from build123d import *

# Parameters (mm, degrees)
SKETCH1_R           = 25
BOSS_EXTRUDE1_DEPTH = 17
CIRPATTERN1_COUNT   = 3
SKETCH14_W          = 15.649879363
SKETCH14_H          = 14
CUT_EXTRUDE2_DEPTH  = 17.25
CUT_EXTRUDE3_DEPTH  = 15
SKETCH16_R          = 2
SKETCH16_R_2        = 1
BOSS_EXTRUDE2_DEPTH = 3


with BuildPart() as part:
    # Sketch1 → Boss-Extrude1 (new body)
    with BuildSketch(Plane.XY):
        Circle(SKETCH1_R)
    extrude(amount=BOSS_EXTRUDE1_DEPTH)

    # Sketch12 → Ø3.0mm Dowel Hole1 (revolve, cut)
    with BuildSketch(Plane(origin=(0, 21, 0), x_dir=(0, 1, 0), z_dir=(1, 0, 0))):
        Polygon((0, 0), (0, 5.901290929), (1.5, 5), (1.5, 0), align=None)
    f_3_0mm_dowel_hole1 = revolve(axis=Axis((0, 21, -6.35), (0, 0, 1)), mode=Mode.SUBTRACT)

    # CirPattern1: Ø3.0mm Dowel Hole1 ×3 about axis
    cirpattern1_axis = Axis((0, 0, 0), (0, 0, 1))
    for i in range(1, CIRPATTERN1_COUNT):
        add(f_3_0mm_dowel_hole1.rotate(cirpattern1_axis, i * 360 / CIRPATTERN1_COUNT), mode=Mode.SUBTRACT)

    # Sketch14 → Cut-Extrude2 (cut)
    with BuildSketch(Plane(origin=(0, -25, 0), x_dir=(-1, 0, 0), z_dir=(0, -1, 0))):
        with Locations((-0.842506508, -8.397851159)):
            Rectangle(SKETCH14_W, SKETCH14_H)
    extrude(amount=-CUT_EXTRUDE2_DEPTH, mode=Mode.SUBTRACT)

    # Sketch15 → Cut-Extrude3 (cut)
    with BuildSketch(Plane(origin=(0, 0, 0), x_dir=(-1, 0, 0), z_dir=(0, 0, -1))):
        with BuildLine():
            ThreePointArc((-3.981818088, 20.619047619), (0, 17), (3.981818088, 20.619047619))
            ThreePointArc((3.981818088, 20.619047619), (18.186533479, 10.5), (19.847528084, -6.861168192))
            ThreePointArc((19.847528084, -6.861168192), (14.722431864, -8.5), (15.865709996, -13.757879427))
            ThreePointArc((15.865709996, -13.757879427), (0, -21), (-15.865709996, -13.757879427))
            ThreePointArc((-15.865709996, -13.757879427), (-14.722431864, -8.5), (-19.847528084, -6.861168192))
            ThreePointArc((-19.847528084, -6.861168192), (-18.186533479, 10.5), (-3.981818088, 20.619047619))
        make_face()
    extrude(amount=-CUT_EXTRUDE3_DEPTH, mode=Mode.SUBTRACT)

    # Sketch16 → Boss-Extrude2 (add)
    with BuildSketch(Plane(origin=(0, 0, 15), x_dir=(-1, 0, 0), z_dir=(0, 0, -1))):
        with Locations((-7, 8.038832814)):
            Circle(SKETCH16_R)
        with Locations((-7, 8.038832814)):
            Circle(SKETCH16_R_2, mode=Mode.SUBTRACT)
        with Locations((7, 8.038832814)):
            Circle(SKETCH16_R)
        with Locations((7, 8.038832814)):
            Circle(SKETCH16_R_2, mode=Mode.SUBTRACT)
    extrude(amount=BOSS_EXTRUDE2_DEPTH)


solid = part.part
Check sheet for the modelled part. Datum: model origin and axes. Units: mm. A direction names the side the tool comes from. Round coordinates to 2 decimals unless told otherwise and drop trailing zeros. Loops run counter-clockwise (first coordinate to the right, second up) from the corner with the lowest first, then second, coordinate; pieces in that order, holes last. Notation, with made-up numbers: (-33.5, 74.5) - (-14.5, 74.5) arc R19 cw to (-14.5, 90.5) - close; hole circle Ø6 at (-35, 46). An arc over 180 degrees is marked (long way). Answer as CSV lines item,"result". Start each with the question number.
Item 1: Release check for a two-part mould opening along X. For faces 1 (the conical face through (-0.078, 21.248, 5.745)), 2 (the cylindrical face through (-3.255, 24.787, 8.381)) record: +X half, -X half, draft (parallel to the pull), parting line (faces both ways), or undercut.
Item 2: Section check C-C (x = -10.5). Record the boundary of the cut face in (y, z).
Item 3: Section check D-D (y = 18). Record the boundary of the cut face in (x, z), and give its area (3 significant figures).
Item 4: Set-up check for faces 3 (the flat face through (-6, 9, 12)), 4 (the flat face through (1, -16, 15.398)): record each of +Z, -Z, +X, -X, +Y, -Y from which the full face is reachable in a straight line by a thin tool's end or side.
Item 5: Section check B-B (x = 2.5). Record the boundary of the cut face in (y, z), and give its area (3 significant figures).
Item 6: Depth check by flat-ended pin: P1, Ø2.5, axis at x = 7, y = 8.04, coming from the -Z side; P2, Ø4, axis at x = -10, y = 11, coming from the -Z side; P3, Ø1.5, axis at y = 16.5, z = 5.5, coming from the +X side. Enter the tip coordinate at first touch or a pass-through.
Item 7: Section check A-A (y = 0). Record the boundary of the cut face in (x, z), and give its area (3 significant figures).
Item 8: Scan lines: line 1 (X direction, y = -10.5, z = 1.85); line 2 (Y direction, x = 14.5, z = 3); line 3 (X direction, y = -9.5, z = 3). Record each from-to range of solid material in increasing order. Write a range as [from, to].
Report:
1,face 1,"undercut"
1,face 2,"parting line"
2,outline,"(-22.69, 0) - (-18.19, 0) - (-18.19, 15) - (18.19, 15) - (18.19, 0) - (22.69, 0) - (22.69, 17) - (-22.69, 17) - close"
3,outline,"(-17.35, 0) - (-10.82, 0) - (-10.82, 15) - (-2.65, 15) - (-2.65, 0) - (2.65, 0) - (2.65, 15) - (10.82, 15) - (10.82, 0) - (17.35, 0) - (17.35, 17) - (-17.35, 17) - close"
3,area,"345 mm2"
4,face 3,"-Z"
4,face 4,"-Y"
5,outline,"(-24.87, 0) - (-20.85, 0) - (-20.85, 1.4) - (-24.87, 1.4) - close; (-24.87, 15.4) - (-7.75, 15.4) - (-7.75, 15) - (17.88, 15) - (17.88, 0) - (24.87, 0) - (24.87, 17) - (-24.87, 17) - close"
5,area,"203 mm2"
6,P1,"stops at z = 12"
6,P2,"stops at z = 15"
6,P3,"stops at x = 19.41"
7,outline,"(-25, 0) - (-21, 0) - (-21, 15) - (21, 15) - (21, 0) - (25, 0) - (25, 17) - (-25, 17) - close"
7,area,"220 mm2"
8,line 1,"x = [-22.69, -19.69], [-16.69, -14.19], [14.19, 16.69], [19.69, 22.69]"
8,line 2,"y = [-20.37, -15.19], [-12.05, -8.95], [15.19, 20.37]"
8,line 3,"x = [-23.12, -19.3], [-17.07, -14.31], [14.31, 17.07], [19.3, 23.12]"
